```python
from build123d import *

# Parameters (mm, degrees)
F0_W     = 77
F0_H     = 97
F0_R     = 6.375
F1_DEPTH = 3
F2_R     = 10
F2_R_2   = 6.375
F3_DEPTH = 3
F4_W     = 77
F4_H     = 2.929018
F5_DEPTH = 5
F6_R     = 5


with BuildPart() as f1:
    # F0 (on Front) → F1 (new body)
    with BuildSketch(Plane.XZ):
        Rectangle(F0_W, F0_H)
        with Locations((-25.5, 22.5)):
            Circle(F0_R, mode=Mode.SUBTRACT)
    extrude(amount=-F1_DEPTH)

    # F2 (on face) → F3 (join)
    with BuildSketch(Plane.XZ):
        with Locations((-25.5, 22.5)):
            Circle(F2_R)
        with Locations((-25.5, 22.5)):
            Circle(F2_R_2, mode=Mode.SUBTRACT)
    extrude(amount=F3_DEPTH)

    # F4 (on face) → F5 (join)
    with BuildSketch(Plane.XZ):
        Polygon((-38.5, 37.005685), (-38.5, 35.700995), (-38.5, 34.099021), (38.5, 34.099021), (38.5, 35.700995), (38.5, 37.005685), align=None)
        with Locations((0, -18.43647)):
            Rectangle(F4_W, F4_H)
    extrude(amount=F5_DEPTH)

    # F6
    f6_edges = [f1.edges().sort_by_distance(p)[0] for p in [
        (38.5, 1.5, 48.5),
        (-38.5, 1.5, 48.5),
        (38.5, 1.5, -48.5),
        (-38.5, 1.5, -48.5),
    ]]
    fillet(f6_edges, radius=F6_R)


solid = f1.part
```
Model file for the job. Use its own axes, mm. A direction names the side the tool comes from. Give positions to 0.01 mm unless a question says otherwise; leave off trailing zeros. Loops run counter-clockwise (first coordinate to the right, second up) from the corner with the lowest first, then second, coordinate; pieces in that order, holes last. Notation, with made-up numbers: (-22.75, 55) -> (16.25, 55) arc R14 ccw to (16.25, 59) -> close; hole circle Ø11 at (7, 27). An arc over 180 degrees is marked (long way). Write each question's results on one line, items separated by ' | '.
(1) Cut at A-A on x = -25.5. List the corners of the cut face in (y, z) (3 decimals), and give its area (3 significant figures).
Geometry results:
outline: (-5, -19.901) -> (0, -19.901) -> (0, -48.5) -> (3, -48.5) -> (3, 16.125) -> (-3, 16.125) -> (-3, 12.5) -> (0, 12.5) -> (0, -16.972) -> (-5, -16.972) -> close; (-5, 34.099) -> (0, 34.099) -> (0, 32.5) -> (-3, 32.5) -> (-3, 28.875) -> (3, 28.875) -> (3, 48.5) -> (0, 48.5) -> (0, 37.006) -> (-5, 37.006) -> close | area: 304 mm²
(2) Probe line 1 along Z through (x, y) = (-25.5, -1.05) (3 decimals); line 2 along Z through (x, y) = (-2.5, -4); line 3 along Z through (x, y) = (-25.5, 1.2) (3 decimals). List the from-to ranges inside material, lowest first.
Geometry results:
line 1: z = -19.901 to -16.972, 12.5 to 16.125, 28.875 to 32.5, 34.099 to 37.006 | line 2: z = -19.9 to -16.97, 34.1 to 37.01 | line 3: z = -48.5 to 16.125, 28.875 to 48.5
(3) Cut at C-C on x = 1. List the corners of the cut face in (y, z), and give its area (3 significant figures).
Geometry results:
outline: (-5, -19.9) -> (0, -19.9) -> (0, -48.5) -> (3, -48.5) -> (3, 48.5) -> (0, 48.5) -> (0, 37.01) -> (-5, 37.01) -> (-5, 34.1) -> (0, 34.1) -> (0, -16.97) -> (-5, -16.97) -> close | area: 320 mm²
(4) Pull direction Z, two halves, no side cores. Call faces 6 (the flat face through (-38.5, 1, 0)), 7 (the cylindrical face through (-37.07, 1.52, 47)), 8 (the flat face through (-1, -2, 34.099)): released by +Z, released by -Z, zero draft, split by the parting line, or undercut.
Geometry results:
face 6: zero draft | face 7: released by +Z | face 8: undercut
(5) Tool access for faces 1 (the flat face through (-1, 0, -34)), 2 (the flat face through (-1, -5, -18)), 3 (the flat face through (-1, 0, 43)), 4 (the flat face through (-1, 3, 1)), 5 (the flat face through (-1, -2, -16.972)): list every direction of +Z, -Z, +X, -X, +Y, -Y with a clear straight run to the whole face (end or side of a thin tool).
Geometry results:
face 1: -Z, +X, -X, -Y | face 2: +Z, -Z, +X, -X, -Y | face 3: +Z, +X, -X, -Y | face 4: +Z, -Z, +X, -X, +Y | face 5: +X, -X, -Y
(6) Cut at B-B on z = 22.5. List the corners of the cut face in (x, y) (3 decimals), and give its area (4 significant figures).
Geometry results:
outline: (-38.5, 0) -> (-35.5, 0) -> (-35.5, -3) -> (-31.875, -3) -> (-31.875, 3) -> (-38.5, 3) -> close; (-19.125, -3) -> (-15.5, -3) -> (-15.5, 0) -> (38.5, 0) -> (38.5, 3) -> (-19.125, 3) -> close | area: 214.5 mm²
(7) Cut at D-D on z = -4. List the corners of the cut face in (x, y).
Geometry results:
outline: (-38.5, 0) -> (38.5, 0) -> (38.5, 3) -> (-38.5, 3) -> close
(8) Flat gauge pins, fed straight in: pin 1 Ø1.5 at (x, y) = (16, -2) entering from -Z; pin 2 Ø9 at (x, z) = (13.5, 42.5) entering from -Y; pin 3 Ø1.5 at (x, y) = (-12.5, -3.5) entering from +Z. Where does each tip first touch, or does it go through?
Geometry results:
pin 1: stops at z = -19.9 | pin 2: stops at y = 0 | pin 3: stops at z = 37.01
